```python
from build123d import *

# Parameters (mm, degrees)
F1_DEPTH  = 10
F2_R      = 3
F3_R      = 1.5
F4_DEPTH  = 10.001
F5_R      = 2
F6_DEPTH  = 8
F7_R      = 3
F8_DEPTH  = 6
F9_R      = 4
F10_DEPTH = 4
F11_R     = 3
F12_R     = 2
F13_DEPTH = 4.001
F14_R     = 3
F15_R     = 0.5


with BuildPart() as f1:
    # F0 (on Top) → F1 (new body)
    with BuildSketch(Plane.XY):
        Polygon((14, 12.5), (4, 12.5), (-4, 12.5), (-4, -2.5), (-14, -2.5), (-14, -12.5), (-4, -12.5), (4, -12.5), (4, 8.5), (14, 8.5), align=None)
    extrude(amount=F1_DEPTH)

    # F2
    f2_edges = [f1.edges().sort_by_distance(p)[0] for p in [
        (-4, 12.5, 5),
        (4, -12.5, 5),
    ]]
    fillet(f2_edges, radius=F2_R)

    # F3 (on face) → F4 (cut, through all)
    with BuildSketch(Plane(origin=(0, 0, 0), x_dir=(1, 0, 0), z_dir=(0, 0, -1))):
        with Locations((-9, 7.5)):
            Circle(F3_R)
    extrude(amount=-F4_DEPTH, mode=Mode.SUBTRACT)

    # F5 (on face) → F6 (cut)
    with BuildSketch(Plane(origin=(0, 0, 0), x_dir=(1, 0, 0), z_dir=(0, 0, -1))):
        with Locations((-9, 7.5)):
            Circle(F5_R)
    extrude(amount=-F6_DEPTH, mode=Mode.SUBTRACT)

    # F7 (on face) → F8 (cut)
    with BuildSketch(Plane(origin=(0, 0, 0), x_dir=(1, 0, 0), z_dir=(0, 0, -1))):
        with Locations((-9, 7.5)):
            Circle(F7_R)
    extrude(amount=-F8_DEPTH, mode=Mode.SUBTRACT)

    # F9 (on face) → F10 (cut)
    with BuildSketch(Plane(origin=(0, 0, 0), x_dir=(1, 0, 0), z_dir=(0, 0, -1))):
        with Locations((-9, 7.5)):
            Circle(F9_R)
    extrude(amount=-F10_DEPTH, mode=Mode.SUBTRACT)

    # F11
    f11_edges = [f1.edges().sort_by_distance(p)[0] for p in [
        (-14, -2.5, 5),
        (-14, -12.5, 5),
    ]]
    fillet(f11_edges, radius=F11_R)

    # F12 (on face) → F13 (cut, through all)
    with BuildSketch(Plane.XZ.offset(-8.5)):
        with Locations((9, 5)):
            Circle(F12_R)
    extrude(amount=-F13_DEPTH, mode=Mode.SUBTRACT)

    # F14
    f14_edges = [f1.edges().sort_by_distance(p)[0] for p in [
        (14, 10.5, 0),
        (14, 10.5, 10),
    ]]
    fillet(f14_edges, radius=F14_R)

    # F15
    f15_edges = [f1.edges().sort_by_distance(p)[0] for p in [
        (4, 8.5, 5),
        (-4, -2.5, 5),
    ]]
    fillet(f15_edges, radius=F15_R)


solid = f1.part
```
Build history of the part. All positions in model axes, mm. A direction names the side the tool comes from. Give positions to 0.01 mm unless a question says otherwise; leave off trailing zeros. Loops run counter-clockwise (first coordinate to the right, second up) from the corner with the lowest first, then second, coordinate; pieces in that order, holes last.
1) Two-plate mould, pull along Y, no slides. Class faces 1 (the face through (11.3, 8.5, 4.9)), 2 (the face through (-11.4, -5.7, 5)), 3 (the face through (-8, -2.5, 5)): released by +Y, released by -Y, zero draft, split by the parting line, or undercut.
Values follow:
face 1: released by -Y
face 2: undercut
face 3: released by +Y
2) Band-saw the part on C-C on x = 9. List the corners of the cut face in (y, z).
Values follow:
outline: (8.5, 0) - (12.5, 0) - (12.5, 3) - (8.5, 3) - close; (8.5, 7) - (12.5, 7) - (12.5, 10) - (8.5, 10) - close
3) Band-saw the part on A-A on z = 5. List the corners of the cut face in (x, y), then the cut area to 3 significant figures.
Values follow:
outline: (-14, -9.5) arc R3 ccw to (-11, -12.5) - (1, -12.5) arc R3 ccw to (4, -9.5) - (4, 8) arc R0.5 cw to (4.5, 8.5) - (7, 8.5) - (7, 12.5) - (-1, 12.5) arc R3 ccw to (-4, 9.5) - (-4, -2) arc R0.5 cw to (-4.5, -2.5) - (-11, -2.5) arc R3 ccw to (-14, -5.5) - close; (11, 8.5) - (14, 8.5) - (14, 12.5) - (11, 12.5) - close; hole circle Ø6 at (-9, -7.5)
area: 288 mm2
4) Drop flat-ended pins along their axis: P1, Ø4, axis at y = 1, z = 1.5, coming from the +X side; P2, Ø5, axis at x = -9, y = -7.5, coming from the +Z side; P3, Ø5, axis at x = 9, z = 5.5, coming from the -Y side; P4, Ø5.5, axis at x = -9, y = -7.5, coming from the -Z side. Give the stop position or say it passes through.
Values follow:
P1: stops at x = 4
P2: stops at z = 10
P3: stops at y = 8.5
P4: stops at z = 6
5) Band-saw the part on D-D on y = 10. List the corners of the cut face in (x, z), then the cut area to 3 significant figures.
Values follow:
outline: (-3.96, 0) - (11, 0) arc R3 ccw to (14, 3) - (14, 7) arc R3 ccw to (11, 10) - (-3.96, 10) - close; hole circle Ø4 at (9, 5)
area: 163 mm2
6) Probe line 1 along Y through (x, z) = (-9, 7.6); line 2 along X through (y, z) = (-7.5, 7.5); line 3 along Y through (x, z) = (-9, 9.1). List the from-to ranges inside material, lowest first.
Values follow:
line 1: y = -12.5 to -9.5, -5.5 to -2.5
line 2: x = -14 to -11, -7 to 4
line 3: y = -12.5 to -9, -6 to -2.5
7) 3-axis set-ups, long thin cutter, end or side, ignore diameter. For faces 4 (the face through (4, -1, 5)), 5 (the face through (14, 10, 5)), 6 (the face through (-4, 4, 5)), 7 (the face through (-9, -10, 6)), 8 (the face through (1, 0, 0)): which of +Z, -Z, +X, -X, +Y, -Y reach the whole face in a straight line?
Values follow:
face 4: +Z, -Z, +X, -Y
face 5: +Z, -Z, +X, +Y, -Y
face 6: +Z, -Z, -X, +Y
face 7: -Z
face 8: -Z, +X, -X, +Y, -Y
8) Band-saw the part on B-B on y = -7.5. List the corners of the cut face in (x, z), then the cut area to 3 significant figures.
Values follow:
outline: (-14, 0) - (-13, 0) - (-13, 4) - (-12, 4) - (-12, 6) - (-11, 6) - (-11, 8) - (-10.5, 8) - (-10.5, 10) - (-14, 10) - close; (-7.5, 8) - (-7, 8) - (-7, 6) - (-6, 6) - (-6, 4) - (-5, 4) - (-5, 0) - (4, 0) - (4, 10) - (-7.5, 10) - close
area: 122 mm2
